Read the model definition and answer for the solid it produces. Units are mm, in the model's axes. A direction names the side the tool comes from. Coordinates: 2 decimals unless noted, no trailing zeros. Write each loop counter-clockwise with the first axis right and the second up, starting at its lowest first coordinate (ties: lowest second). Pieces come first, ordered by that corner, then holes.
(1) Straight lines are drawn through the part: line 1 along Z through (x, y) = (8.5, 3); line 2 along X through (y, z) = (4.25, 2). For each, find the intervals that lie inside material, in ascending order.
(2) Given pin 1 (12 mm diameter, centred on x = 16.5, y = -9.5, fed in from +Z); pin 2 (4 mm diameter, centred on y = 7.5, z = 9.5, fed in from +X), each flat-ended and moving along its own axis, determine where each tip first touches the part or whether it passes through.
(3) The part is cut by section A-A, the plane x = 11.25. Determine the outline of the cut face in (y, z), and give its area (3 significant figures).
(4) The part is cut by section C-C, the plane y = -5.75. Determine the outline of the cut face in (x, z), and give its area (3 significant figures).
(5) The part is cut by section D-D, the plane x = 5. Determine the outline of the cut face in (y, z).
(6) Determine the mould class of faces 1 (the flat face through (12, 3, 0)), 2 (the flat face through (6, -12.7, 1)), 3 (the cylindrical face through (0.773, 1.408, 10.998)), 4 (the flat face through (11, 3, 1.524)) for opening direction Z: pulls with the +Z half, pulls with the -Z half, needs draft (parallel to the pull), parting line crosses it, or undercut.
(7) Which of the six approach directions +Z, -Z, +X, -X, +Y, -Y give full straight-line access (tool end or side, diameter ignored) to faces 5 (the flat face through (12, 2.083, 1)), 6 (the flat face through (6, 12.7, 1)), 7 (the flat face through (1.524, 0, 12))?
(8) The part is cut by section B-B, the plane y = 0. Determine the outline of the cut face in (x, z), and give its area (3 significant figures).
```python
from build123d import *

# Parameters (mm, degrees)
EXTRUDE_THIN1_START = -12.7
EXTRUDE_THIN1_DEPTH = 25.4
SKETCH4_R           = 2.0828
EXTRUDE3_DEPTH      = 29.836691705
CUT_EXTRUDE1_DEPTH  = 30.868634259


# Read off the part's stored shape, not the designer's step: Extrude-Thin1
with BuildPart() as part:
    # Extrude-Thin1 outline → Extrude-Thin1 (new body)
    with BuildSketch(Plane(origin=(0, 0, 0), x_dir=(1, 0, 0), z_dir=(0, 1, 0)).offset(EXTRUDE_THIN1_START)):
        with BuildLine():
            Line((2.286, -1.524), (20.6375, -1.524))
            Line((20.6375, -1.524), (20.6375, 0))
            Line((20.6375, 0), (2.286, 0))
            ThreePointArc((2.286, 0), (0.669553898, -0.669553898), (0, -2.286))
            Line((0, -2.286), (0, -17.4625))
            Line((0, -17.4625), (1.524, -17.4625))
            Line((1.524, -17.4625), (1.524, -2.286))
            ThreePointArc((1.524, -2.286), (1.747184633, -1.747184633), (2.286, -1.524))
        make_face()
    extrude(amount=EXTRUDE_THIN1_DEPTH)

    # Sketch4 → Extrude3 (cut, through all)
    with BuildSketch(Plane(origin=(1.524, 0, 0), x_dir=(0, 0, -1), z_dir=(1, 0, 0))):
        with Locations((-9.4625, 0)):
            Circle(SKETCH4_R)
    extrude(amount=-EXTRUDE3_DEPTH, mode=Mode.SUBTRACT)

    # Sketch6 → Cut-Extrude1 (cut, through all)
    with BuildSketch(Plane.XY):
        with BuildLine():
            Line((7.6375, 2.0828), (15.6375, 2.0828))
            ThreePointArc((15.6375, 2.0828), (17.7203, 0), (15.6375, -2.0828))
            Line((15.6375, -2.0828), (7.6375, -2.0828))
            ThreePointArc((7.6375, -2.0828), (5.5547, 0), (7.6375, 2.0828))
        make_face()
    extrude(amount=CUT_EXTRUDE1_DEPTH, mode=Mode.SUBTRACT)


solid = part.part
```
Computed:
1. line 1: z = 0 to 1.52
1. line 2: x = 0.02 to 1.58
2. pin 1: stops at z = 1.52
2. pin 2: stops at x = 1.52
3. outline: (-12.7, 0) - (-2.08, 0) - (-2.08, 1.52) - (-12.7, 1.52) - close; (2.08, 0) - (12.7, 0) - (12.7, 1.52) - (2.08, 1.52) - close
3. area: 32.4 mm2
4. outline: (0, 2.29) arc R2.29 ccw to (2.29, 0) - (20.64, 0) - (20.64, 1.52) - (2.29, 1.52) arc R0.76 cw to (1.52, 2.29) - (1.52, 17.46) - (0, 17.46) - close
4. area: 54.7 mm2
5. outline: (-12.7, 0) - (12.7, 0) - (12.7, 1.52) - (-12.7, 1.52) - close
6. face 1: pulls with the -Z half
6. face 2: needs draft
6. face 3: undercut
6. face 4: pulls with the +Z half
7. face 5: +Z, -Z
7. face 6: +Z, -Z, +X, -X, +Y
7. face 7: +Z, +X, +Y, -Y
8. outline: (0, 2.29) arc R2.29 ccw to (2.29, 0) - (5.55, 0) - (5.55, 1.52) - (2.29, 1.52) arc R0.76 cw to (1.52, 2.29) - (1.52, 7.38) - (0, 7.38) - close; (0, 11.55) - (1.52, 11.55) - (1.52, 17.46) - (0, 17.46) - close; (17.72, 0) - (20.64, 0) - (20.64, 1.52) - (17.72, 1.52) - close
8. area: 29.9 mm2
